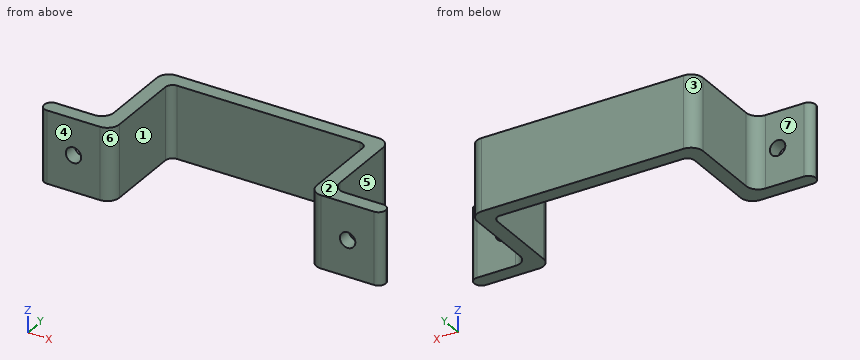
```python
from build123d import *

# Parameters (mm, degrees)
BOSS_EXTRUDE1_DEPTH = 7.5
SKETCH2_R           = 1.6
CUT_EXTRUDE2_DEPTH  = 42.191625362
FILLET1_R           = 2.5
FILLET2_R           = 1.5


with BuildPart() as part:
    # Sketch1 → Boss-Extrude1 (new, symmetric)
    with BuildSketch(Plane.XY):
        Polygon((-23.5, 12.75), (23.5, 12.75), (23.5, -6.75), (35.5, -6.75), (35.5, -9.75), (20.5, -9.75), (20.5, 9.75), (-20.5, 9.75), (-20.5, -9.75), (-35.5, -9.75), (-35.5, -6.75), (-23.5, -6.75), align=None)
    extrude(amount=BOSS_EXTRUDE1_DEPTH, both=True)

    # Sketch2 → Cut-Extrude2 (cut, through all)
    with BuildSketch(Plane(origin=(0, -6.75, 0), x_dir=(1, 0, 0), z_dir=(0, 1, 0))):
        with Locations(Location((-28.5, 0, 0), (0, 0, 270))):
            Circle(SKETCH2_R)
        with Locations(Location((28.5, 0, 0), (0, 0, 270))):
            Circle(SKETCH2_R)
    extrude(amount=-CUT_EXTRUDE2_DEPTH, mode=Mode.SUBTRACT)

    # Fillet1
    fillet1_edges = [part.edges().sort_by_distance(p)[0] for p in [
        (23.5, -6.75, 0),
        (20.5, -9.75, 0),
        (-20.5, -9.75, 0),
        (-23.5, -6.75, 0),
        (-23.5, 12.75, 0),
        (23.5, 12.75, 0),
    ]]
    fillet(fillet1_edges, radius=FILLET1_R)

    # Fillet2
    fillet2_edges = [part.edges().sort_by_distance(p)[0] for p in [
        (35.5, -6.75, 0),
        (35.5, -9.75, 0),
        (20.5, 9.75, 0),
        (-20.5, 9.75, 0),
        (-35.5, -9.75, 0),
        (-35.5, -6.75, 0),
    ]]
    fillet(fillet2_edges, radius=FILLET2_R - 0.0001)  # a hair under: the kernel refuses the full size


solid = part.part
```
Geometry: final body of the model. Coordinates: model frame, mm. Face numbers are marked on the shaded views. A direction names the side the tool comes from. Give positions to 0.01 mm unless a question says otherwise; leave off trailing zeros. Loops run counter-clockwise (first coordinate to the right, second up) from the corner with the lowest first, then second, coordinate; pieces in that order, holes last. Notation, with made-up numbers: (68.5, -5.5) -> (107.5, -5.5) arc R11 ccw to (107.5, 14.5) -> close; hole circle Ø2 at (-34.75, -36.75). An arc over 180 degrees is marked (long way). Use one line per item in the form item = value.
Item 1: Section query A-A on z = 0. Give the number of separate pieces and of enclosed holes in the cut face, and give its area (3 significant figures).
A:
separate_pieces = 3
enclosed_holes = 0
area = 307 mm^2
Item 2: Section query B-B on x = -28.5. Output: boundary loops of the cut face in (y, z).
A:
outline = (-9.75, -7.5) -> (-6.75, -7.5) -> (-6.75, -1.6) -> (-9.75, -1.6) -> close; (-9.75, 1.6) -> (-6.75, 1.6) -> (-6.75, 7.5) -> (-9.75, 7.5) -> close
Item 3: Access query for the marked faces 4, 5, 6 and 7. Directions: +Z, -Z, +X, -X, +Y, -Y. A direction counts if a zero-diameter tool reaches every point of the face in a straight line with its end or side. Return the directions, or none.
A:
face_4 = +Z, -Z, +X, -X, -Y
face_5 = +Z, -Z, +X, +Y
face_6 = +Z, -Z, -Y
face_7 = +Z, -Z, -X, +Y
Item 4: Pin query (flat end, axial travel): P1, Ø7, axis at y = 5, z = -3, coming from the -X side; P2, Ø10, axis at x = -14, y = 1, coming from the -Z side; P3, Ø6.5, axis at x = -31, z = 1.5, coming from the +Y side; P4, Ø3, axis at y = 4, z = 5.5, coming from the +X side. Return the tip coordinate at first contact, or that it passes through.
A:
P1 = -23.5
P2 = through
P3 = -6.75
P4 = 23.5
Item 5: Section query D-D on x = 11. Output: boundary loops of the cut face in (y, z).
A:
outline = (9.75, -7.5) -> (12.75, -7.5) -> (12.75, 7.5) -> (9.75, 7.5) -> close
Item 6: Line query: probe 1 along X at (y, z) = (-0.5, 2.5); probe 2 along X at (y, z) = (-7.85, 0); probe 3 along X at (y, z) = (-8.5, 0). Output: solid intervals per line, ascending.
A:
probe_1 = -23.5 to -20.5, 20.5 to 23.5
probe_2 = -35.45 to -30.1, -26.9 to -20.57, 20.57 to 26.9, 30.1 to 35.45
probe_3 = -35.48 to -30.1, -26.9 to -20.83, 20.83 to 26.9, 30.1 to 35.48
Item 7: Draft query along X for the marked faces 1, 2 and 3. Return one class per face: pulls with the +X half, pulls with the -X half, needs draft (parallel to the pull), parting line crosses it, or undercut.
A:
face_1 = undercut
face_2 = needs draft
face_3 = pulls with the -X half
